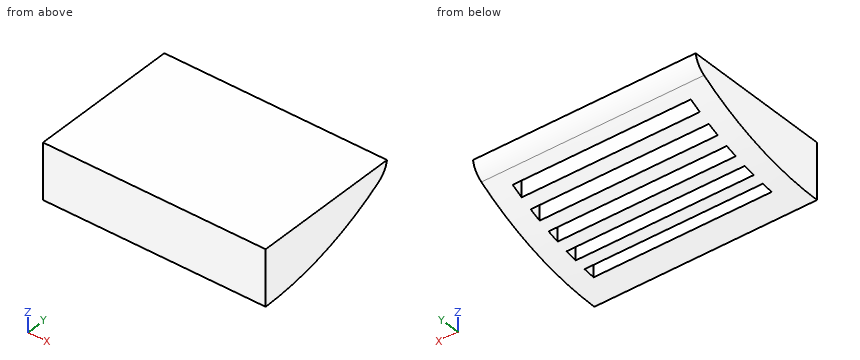
```python
from build123d import *

# Parameters (mm, degrees)
F0_W        = 10
F0_H        = 7.142
F1_DEPTH    = 2.5
F3_DEPTH    = 10.001
F4_T1_DEPTH = 12.7651557864
F6_W        = 8
F6_H        = 0.5
F7_DEPTH    = 2


# Not quite as in the source:
# - a fillet or chamfer that OpenCascade refuses, or shapes differently, is made with other operations: its cross-section is extruded or revolved along the edge and cut away or added


with BuildPart() as f1:
    # F0 (on Top) → F1 (new body)
    with BuildSketch(Plane.XY):
        with Locations((5, 3.571)):
            Rectangle(F0_W, F0_H)
    extrude(amount=F1_DEPTH)

    # F2 (on face) → F3 (cut, through all)
    with BuildSketch(Plane(origin=(0, 0, 0), x_dir=(0, -1, 0), z_dir=(-1, 0, 0))):
        with BuildLine():
            ThreePointArc((0, 0), (-3.5295320322, 0.5584308586), (-6.75, 2.106987431))
            Line((-6.75, 2.106987431), (-6.75, 12.27143))
            Line((-6.75, 12.27143), (-9.8289949819, -2.3460234515))
            Line((-9.8289949819, -2.3460234515), (0, 0))
        make_face()
    extrude(amount=-F3_DEPTH, mode=Mode.SUBTRACT)

    # F4: fillet of radius 1 on 1 edges, made by hand

    # F4_s2 → F4_t1 (cut)
    with BuildSketch(Plane.YZ.offset(-1.3825778932)):
        with BuildLine():
            ThreePointArc((6.75, 2.5), (6.5929931831, 2.1031503004), (6.2848187014, 1.8079058028))
            ThreePointArc((6.2848187014, 1.8079058028), (6.5190889746, 1.9548341876), (6.75, 2.106987431))
            Line((6.75, 2.106987431), (6.75, 2.5))
        make_face()
    extrude(amount=F4_T1_DEPTH, mode=Mode.SUBTRACT)

    # F6 (on offset) → F7 (cut)
    with BuildSketch(Plane.XY):
        with Locations((5, 4.5299213873)):
            Rectangle(F6_W, F6_H)
        with Locations((5, 3.5299213873)):
            Rectangle(F6_W, F6_H)
        with Locations((5, 2.5299213873)):
            Rectangle(F6_W, F6_H)
        with Locations((5, 1.5299213873)):
            Rectangle(F6_W, F6_H)
        with Locations((5, 5.5299213873)):
            Rectangle(F6_W, F6_H)
    extrude(amount=F7_DEPTH, mode=Mode.SUBTRACT)


solid = f1.part
```
Can you work these out from the model? Positions are in its coordinate system, mm. Give positions to 0.01 mm unless a question says otherwise; leave off trailing zeros. Loops run counter-clockwise (first coordinate to the right, second up) from the corner with the lowest first, then second, coordinate; pieces in that order, holes last. Notation, with made-up numbers: M 1,78 L 33,78 A34 ccw 33,113 Z; hole C 20,62 d3. An arc over 180 degrees is marked long. Answer in a Markdown table with one row per item.
1. Suppose I cut it at A-A on z = 1.7. Write out the boundary of the cut face in (x, y), plus the area to 3 significant figures.
Taken from the geometry:
| item | result |
|---|---|
| outline | M 0,0 L 10,0 L 10,6.1 L 0,6.1 Z; hole M 1,1.28 L 9,1.28 L 9,1.78 L 1,1.78 Z; hole M 1,2.28 L 9,2.28 L 9,2.78 L 1,2.78 Z; hole M 1,3.28 L 9,3.28 L 9,3.78 L 1,3.78 Z; hole M 1,4.28 L 9,4.28 L 9,4.78 L 1,4.78 Z; hole M 1,5.28 L 9,5.28 L 9,5.78 L 1,5.78 Z |
| area | 41.0 mm² |
2. Suppose I cut it at D-D on y = 6.5. Write out the boundary of the cut face in (x, z).
Taken from the geometry:
| item | result |
|---|---|
| outline | M 0,1.99 L 10,1.99 L 10,2.5 L 0,2.5 Z |
3. If I drill on line 1 along Y through (x, z) = (5.75, 0.95); line 2 along Y through (x, z) = (2.25, 0.3); line 3 along Y through (x, z) = (5.5, 0.6), over which ranges is the centre line in solid material (lowest first)?
Taken from the geometry:
| item | result |
|---|---|
| line 1 | y = 0 to 1.28, 1.78 to 2.28, 2.78 to 3.28, 3.78 to 4.28 |
| line 2 | y = 0 to 1.28, 1.78 to 2.28 |
| line 3 | y = 0 to 1.28, 1.78 to 2.28, 2.78 to 3.28 |
4. Suppose I cut it at B-B on x = 4.75. Write out the boundary of the cut face in (y, z).
Taken from the geometry:
| item | result |
|---|---|
| outline | M 0,0 A12.31 ccw 1.28,0.08 L 1.28,2 L 1.78,2 L 1.78,0.15 A12.31 ccw 2.28,0.24 L 2.28,2 L 2.78,2 L 2.78,0.35 A12.31 ccw 3.28,0.48 L 3.28,2 L 3.78,2 L 3.78,0.64 A12.31 ccw 4.28,0.82 L 4.28,2 L 4.78,2 L 4.78,1.02 A12.31 ccw 5.28,1.26 L 5.28,2 L 5.78,2 L 5.78,1.52 A12.31 ccw 6.28,1.81 A1 ccw 6.75,2.5 L 0,2.5 Z |
5. Suppose I cut it at C-C on y = 2. Write out the boundary of the cut face in (x, z).
Taken from the geometry:
| item | result |
|---|---|
| outline | M 0,0.19 L 10,0.19 L 10,2.5 L 0,2.5 Z |
6. For pin 1 Ø0.6 at (x, z) = (3.5, 1.5) entering from +Y; pin 2 Ø4 at (x, y) = (4, 4) entering from -Z; pin 3 Ø1.2 at (x, z) = (6, 1) entering from +Y, each with a flat end and sliding along its axis, tell me the tip position at first contact or that it passes through.
Taken from the geometry:
| item | result |
|---|---|
| pin 1 | stops at y = 6.27 |
| pin 2 | stops at z = 0.19 |
| pin 3 | stops at y = 5.93 |
